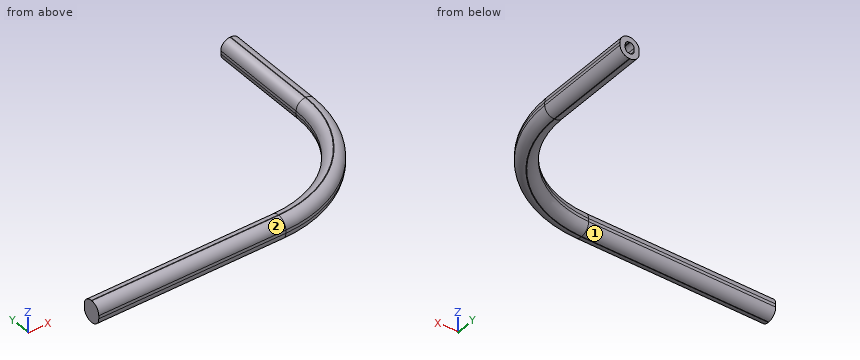
Autodesk Inventor part; units mm, degrees
ref_plane "YZ Plane" through (0, 0, 0) normal (1, 0, 0) x (0, 1, 0)
ref_plane "XZ Plane" through (0, 0, 0) normal (0, 1, 0) x (-1, 0, 0)
ref_plane "XY Plane" through (0, 0, 0) normal (0, 0, 1) x (1, 0, 0)
sketch "Sketch1" plane through (0, 0, 0) normal (0, 0, 1) x (1, 0, 0)
  line L0 (0, 0) -> (95.9616, 0)
  line L1 (0, 0) -> (0, 9.8571)
  line L2 (0, 9.8571) -> (78.8567, 9.8571)
  arc A0 (95.9616, 0) -> (157.7134, 61.7524) centre (95.9616, 61.7517) ccw
  line L3 (78.8567, 9.8571) -> (95.9616, 9.8571)
  arc A1 (95.9616, 9.8571) -> (147.8563, 61.7517) centre (95.9616, 61.7517) ccw
  line L4 (147.8563, 61.7517) -> (147.8563, 112.8865)
  line L5 (147.8563, 112.8865) -> (157.7134, 112.8865)
  line L6 (157.7134, 112.8865) -> (157.7134, 61.7524)
extrude "Extrusion1" add sketch "Sketch1" along normal blind 11.1125
fillet "Fillet1" radius 4.7625 12 edges at (132.6567, 25.0567, 0) (147.8563, 87.3191, 0) (39.4283, 9.8571, 0) (132.6567, 25.0567, 11.1125) (147.8563, 87.3191, 11.1125) (39.4283, 9.8571, 11.1125) (139.6269, 18.0869, 11.1125) (157.7134, 87.3194, 11.1125) (47.9808, 0, 11.1125) (157.7134, 87.3194, 0) (47.9808, 0, 0) (139.6269, 18.0869, 0)
shell "Shell1" thickness 2.667 removed faces 1 at (152.8402, 112.8865, 3.175)
properties part number "pipe2"
Could you check a few things on this model? Use its own coordinates, in mm. Face numbers are marked on the shaded views. A direction names the side the tool comes from. Give positions to 0.01 mm unless a question says otherwise; leave off trailing zeros. Return JSON: item names as keys, results as strings.
1. For pin 1 Ø2 at (x, z) = (116.5, 1) entering from +Y; pin 2 Ø0.5 at (x, z) = (26, 6) entering from +Y; pin 3 Ø1 at (x, z) = (112, 6) entering from +Y, each with a flat end and sliding along its axis, tell me the tip position at first contact or that it passes through.
Answer list:
{"pin 1": "stops at y = 13.24", "pin 2": "stops at y = 9.86", "pin 3": "stops at y = 12.56"}
2. I need wall thicknesses on line 1 (Y direction, x = 95.5, z = 6.5); line 2 (X direction, y = 87, z = 5.25); line 3 (X direction, y = 68, z = 6.75). Which ranges of each line are inside material? Lowest first, please. Write a range as from..to.
Answer list:
{"line 1": "y = 0..2.67, 7.18..9.85", "line 2": "x = 147.86..150.52, 155.05..157.71", "line 3": "x = 147.87..150.56, 155.01..157.7"}
3. On a 3-axis mill with a long thin cutter (end or side, diameter ignored), from which of +Z, -Z, +X, -X, +Y, -Y can I reach the whole of each face in a straight line? I mean the marked faces 1 and 2. Say none if no direction works.
Answer list:
{"face 1": "-Z, -X, +Y", "face 2": "+Z, +X, -X, -Y"}
